```python
from build123d import *

# Parameters (mm, degrees)
F0_W           = 200
F0_H           = 60
F1_DEPTH       = 5
F3_D           = 11
F3_CSINK_D     = 22.4
F3_CSINK_ANGLE = 90
F4_R           = 11


with BuildPart() as f1:
    # F0 (on Top) → F1 (new body)
    with BuildSketch(Plane.XY):
        Rectangle(F0_W, F0_H)
    extrude(amount=F1_DEPTH)

    # F3 (through all)
    with Locations(Plane.XY.offset(5)):
        with Locations((-85, 15), (-25, 15), (25, 15), (-55, -15), (55, -15), (85, 15)):
            CounterSinkHole(F3_D / 2, F3_CSINK_D / 2, counter_sink_angle=F3_CSINK_ANGLE)

    # F4
    f4_edges = [f1.edges().sort_by_distance(p)[0] for p in [
        (-100, 30, 2.5),
        (-100, -30, 2.5),
        (100, -30, 2.5),
        (100, 30, 2.5),
    ]]
    fillet(f4_edges, radius=F4_R)


solid = f1.part
```
Here's how the part is built. I have some questions about the finished solid (model axes, mm). Give positions to 0.01 mm unless a question says otherwise; leave off trailing zeros. Write each loop counter-clockwise with the first axis right and the second up, starting at its lowest first coordinate (ties: lowest second). Pieces come first, ordered by that corner, then holes.
(1) Imagine slicing it at A-A, the plane x = -25. Write out the boundary of the cut face in (y, z), and give its area (3 significant figures).
Output values:
outline: (-30, 0) - (8.8, 0) - (3.8, 5) - (-30, 5) - close; (21.2, 0) - (30, 0) - (30, 5) - (26.2, 5) - close
area: 213 mm2
(2) Imagine slicing it at C-C, the plane y = 15. Write out the boundary of the cut face in (x, z).
Output values:
outline: (-100, 0) - (-91.2, 0) - (-96.2, 5) - (-100, 5) - close; (-78.8, 0) - (-31.2, 0) - (-36.2, 5) - (-73.8, 5) - close; (-18.8, 0) - (18.8, 0) - (13.8, 5) - (-13.8, 5) - close; (31.2, 0) - (78.8, 0) - (73.8, 5) - (36.2, 5) - close; (91.2, 0) - (100, 0) - (100, 5) - (96.2, 5) - close
(3) Thinking about a two-plate mould opening in X: for faces 1 (the face through (-1, 0, 5)), 2 (the face through (60.11, -18.92, 0.24)), 3 (the face through (96.863, 26.692, 2.535)), 4 (the face through (-100, 0, 2)), which applies, pulls with the +X half, pulls with the -X half, needs draft (parallel to the pull), parting line crosses it, or undercut?
Output values:
face 1: needs draft
face 2: undercut
face 3: pulls with the +X half
face 4: pulls with the -X half
(4) If I drill on L1, parallel to X at y = 13, z = 1.1; L2, parallel to X at y = 11.5, z = 4.1; L3, parallel to X at y = -12.5, z = 1.7, over which ranges is the centre line in solid material (lowest first)?
Output values:
L1: x = -100 to -92.02, -77.98 to -32.02, -17.98 to 17.98, 32.02 to 77.98, 92.02 to 100
L2: x = -100 to -94.69, -75.31 to -34.69, -15.31 to 15.31, 34.69 to 75.31, 94.69 to 100
L3: x = -100 to -62.49, -47.51 to 47.51, 62.49 to 100
(5) Imagine slicing it at D-D, the plane y = -15. Write out the boundary of the cut face in (x, z).
Output values:
outline: (-100, 0) - (-61.2, 0) - (-66.2, 5) - (-100, 5) - close; (-48.8, 0) - (48.8, 0) - (43.8, 5) - (-43.8, 5) - close; (61.2, 0) - (100, 0) - (100, 5) - (66.2, 5) - close
(6) Imagine slicing it at B-B, the plane z = 3.6. Write out the boundary of the cut face in (x, y), and give its area (3 significant figures).
Output values:
outline: (-100, -19) arc R11 ccw to (-89, -30) - (89, -30) arc R11 ccw to (100, -19) - (100, 19) arc R11 ccw to (89, 30) - (-89, 30) arc R11 ccw to (-100, 19) - close; hole circle Ø19.6 at (-85, 15); hole circle Ø19.6 at (-55, -15); hole circle Ø19.6 at (-25, 15); hole circle Ø19.6 at (25, 15); hole circle Ø19.6 at (55, -15); hole circle Ø19.6 at (85, 15)
area: 10,100 mm2
